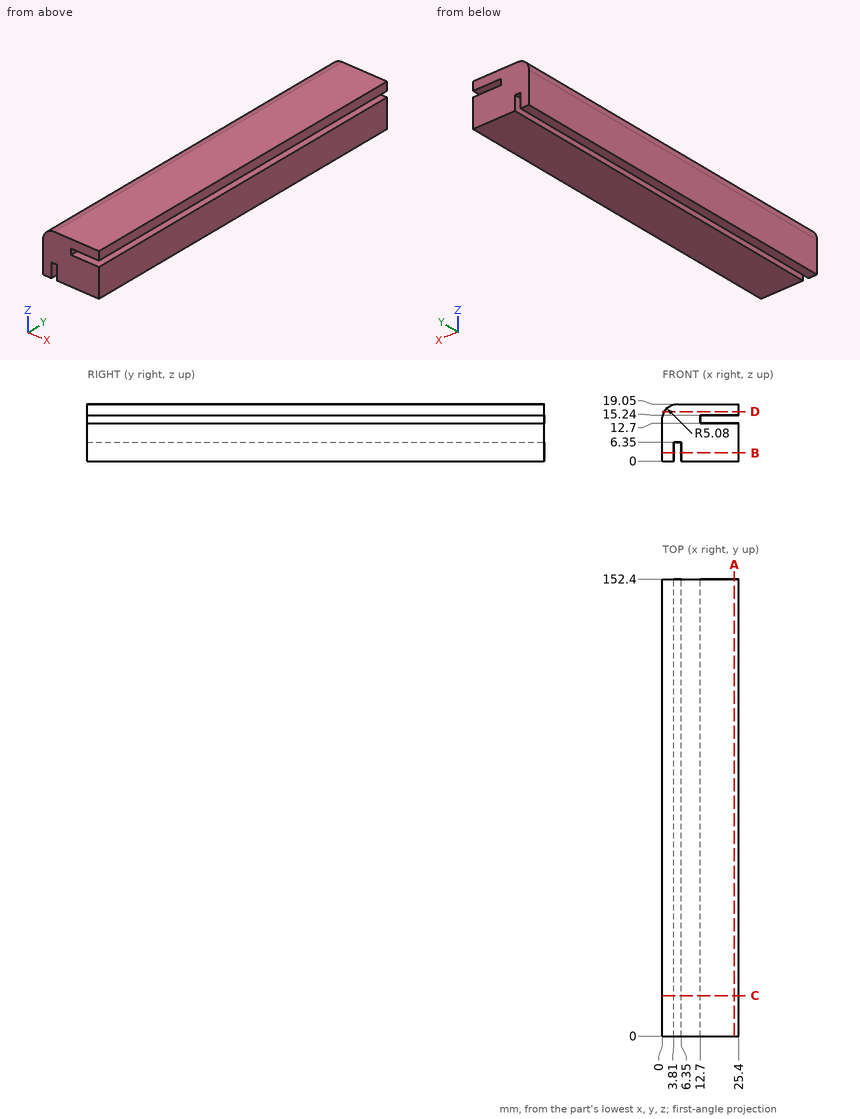
Study the drawing (mm; zero at the part's minimum x, y, z) and answer. Give positions to 0.01 mm unless a question says otherwise; leave off trailing zeros. Loops run counter-clockwise (first coordinate to the right, second up) from the corner with the lowest first, then second, coordinate; pieces in that order, holes last. Notation, with made-up numbers: M -32,33.25 L 26,33.25 A37 cw 26,71.25 Z; hole C 10,89 d2. An arc over 180 degrees is marked long. Use CSV: the item, a comma, the result in double quotes.
1) Given P1, Ø0.8, axis at x = 5, y = 61.5, coming from the -Z side, flat-ended and moving along its own axis, determine where the tip first touches the part or whether it passes through.
Answer:
P1,"z = 6.35"
2) Find section D-D on z = 16.5. Write down the section's boundary in (x, y), plus the area to 3 significant figures.
Answer:
outline,"M 0.67,0 L 25.4,0 L 25.4,152.4 L 0.67,152.4 Z"
area,"3,770 mm^2"
3) Find section B-B on z = 2.75. Write down the section's boundary in (x, y), plus the area to 3 significant figures.
Answer:
outline,"M 0,0 L 3.81,0 L 3.81,152.4 L 0,152.4 Z; M 6.35,0 L 25.4,0 L 25.4,152.4 L 6.35,152.4 Z"
area,"3,480 mm^2"
4) Find section C-C on y = 13.5. Write down the section's boundary in (x, z).
Answer:
outline,"M 0,0 L 3.81,0 L 3.81,6.35 L 6.35,6.35 L 6.35,0 L 25.4,0 L 25.4,12.7 L 12.7,12.7 L 12.7,15.24 L 25.4,15.24 L 25.4,19.05 L 5.08,19.05 A5.08 ccw 0,13.97 Z"
5) Consider L1, parallel to Z at x = 23.5, y = 92.5; L2, parallel to X at y = 77.5, z = 2.75; L3, parallel to X at y = 137.5, z = 13.5. Determine where each line is inside the solid, lowest interval first.
Answer:
L1,"0 to 12.7, 15.24 to 19.05"
L2,"0 to 3.81, 6.35 to 25.4"
L3,"0 to 12.7"
6) Find section A-A on x = 24. Write down the section's boundary in (y, z).
Answer:
outline,"M 0,0 L 152.4,0 L 152.4,12.7 L 0,12.7 Z; M 0,15.24 L 152.4,15.24 L 152.4,19.05 L 0,19.05 Z"
